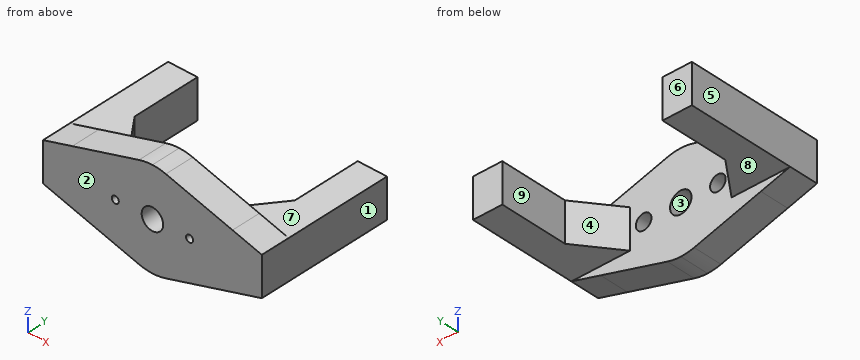
```python
from build123d import *

# Parameters (mm, degrees)
SKETCH1_R               = 25
SKETCH1_R_2             = 1.8
SKETCH1_R_3             = 5.5
BOSS_EXTRUDE1_DEPTH     = 15
SKETCH2_R               = 4
CUT_EXTRUDE1_DEPTH      = 8
SKETCH3_W               = 82
SKETCH3_H               = 50
SKETCH3_R               = 24.5
BOSS_EXTRUDE2_DEPTH     = 15
SKETCH4_W               = 15
SKETCH4_H               = 20
BOSS_EXTRUDE3_DEPTH     = 70
CUT_EXTRUDE2_DEPTH      = 94.064493766
CUT_EXTRUDE2_DEPTH_BACK = 94.064493766
BOSS_EXTRUDE4_DEPTH     = 15
CHAMFER1_SIZE           = 15
CHAMFER1_SIZE2          = 19.905672324


with BuildPart() as part:
    # Sketch1 → Boss-Extrude1 (new body)
    with BuildSketch(Plane(origin=(0, 0, 0), x_dir=(1, 0, 0), z_dir=(0, 1, 0))):
        with Locations(Location((0, 0, 0), (0, 0, 270))):
            Circle(SKETCH1_R)
        with Locations(Location((-19, 0, 0), (0, 0, 270))):
            Circle(SKETCH1_R_2, mode=Mode.SUBTRACT)
        with Locations(Location((19, 0, 0), (0, 0, 90))):
            Circle(SKETCH1_R_2, mode=Mode.SUBTRACT)
        with Locations(Location((0, 0, 0), (0, 0, 270))):
            Circle(SKETCH1_R_3, mode=Mode.SUBTRACT)
    extrude(amount=BOSS_EXTRUDE1_DEPTH)

    # Sketch2 → Cut-Extrude1 (cut)
    with BuildSketch(Plane(origin=(0, 15, 0), x_dir=(1, 0, 0), z_dir=(0, 1, 0))):
        with Locations(Location((-19, 0, 0), (0, 0, 270))):
            Circle(SKETCH2_R)
        with Locations(Location((19, 0, 0), (0, 0, 270))):
            Circle(SKETCH2_R)
    extrude(amount=-CUT_EXTRUDE1_DEPTH, mode=Mode.SUBTRACT)

    # Sketch3 → Boss-Extrude2 (add)
    with BuildSketch(Plane.XZ):
        Rectangle(SKETCH3_W, SKETCH3_H)
        Circle(SKETCH3_R, mode=Mode.SUBTRACT)
    extrude(amount=-BOSS_EXTRUDE2_DEPTH)

    # Sketch4 → Boss-Extrude3 (add)
    with BuildSketch(Plane.XZ):
        with Locations((-48.5, 0)):
            Rectangle(SKETCH4_W, SKETCH4_H)
        with Locations((48.5, 0)):
            Rectangle(SKETCH4_W, SKETCH4_H)
    extrude(amount=-BOSS_EXTRUDE3_DEPTH)

    # Sketch5 → Cut-Extrude2 (cut, two sides: drawn at the far end of the back side and taken through both)
    with BuildSketch(Plane.XZ.offset(-CUT_EXTRUDE2_DEPTH_BACK)):
        Polygon((-41, -25), (-41, -14.285834105), (-56, -10), (-56, -25), align=None)
        with BuildLine():
            ThreePointArc((-2.6e-08, -25), (-3.467621731, -24.758344039), (-6.86820572, -24.03804797))
            Line((-6.86820572, -24.03804797), (-41, -14.285834105))
            Line((-41, -14.285834105), (-41, -25))
            Line((-41, -25), (-2.6e-08, -25))
        make_face()
        Polygon((-56, 25), (-56, 10), (-41, 14.285834105), (-41, 25), align=None)
        with BuildLine():
            Line((-41, 25), (-41, 14.285834105))
            Line((-41, 14.285834105), (-6.86820572, 24.03804797))
            ThreePointArc((-6.86820572, 24.03804797), (-3.467621732, 24.758344038), (-2.8e-08, 25))
            Line((-2.8e-08, 25), (-41, 25))
        make_face()
        with BuildLine():
            Line((41, 25), (-2.8e-08, 25))
            ThreePointArc((-2.8e-08, 25), (3.467621704, 24.758344042), (6.86820572, 24.03804797))
            Line((6.86820572, 24.03804797), (41, 14.285834105))
            Line((41, 14.285834105), (41, 25))
        make_face()
        with BuildLine():
            ThreePointArc((6.86820572, -24.03804797), (3.467621705, -24.758344042), (-2.6e-08, -25))
            Line((-2.6e-08, -25), (41, -25))
            Line((41, -25), (41, -14.285834105))
            Line((41, -14.285834105), (6.86820572, -24.03804797))
        make_face()
        Polygon((41, -14.285834105), (41, -25), (56, -25), (56, -10), align=None)
        Polygon((56, 25), (41, 25), (41, 14.285834105), (56, 10), align=None)
    extrude(amount=CUT_EXTRUDE2_DEPTH + CUT_EXTRUDE2_DEPTH_BACK, mode=Mode.SUBTRACT)

    # Sketch6 → Boss-Extrude4 (add)
    with BuildSketch(Plane.XZ):
        Polygon((-56, 10), (-41, 14.285834105), (-41, -14.285834105), (-56, -10), align=None)
        Polygon((41, 14.285834105), (56, 10), (56, -10), (41, -14.285834105), align=None)
    extrude(amount=-BOSS_EXTRUDE4_DEPTH)

    # Chamfer1
    chamfer1_edges = [part.edges().sort_by_distance(p)[0] for p in [
        (-41, 15, 0),
        (41, 15, 0),
    ]]
    chamfer1_side = [part.faces().sort_by_distance(p)[0] for p in [
        (0, 15, 23.773460151),
    ]]
    chamfer(chamfer1_edges, length=CHAMFER1_SIZE, length2=CHAMFER1_SIZE2, reference=chamfer1_side[0])


solid = part.part
```
Could you check a few things on this model? Use its own coordinates, in mm. Face numbers are marked on the shaded views. A direction names the side the tool comes from. Coordinates: 2 decimals unless noted, no trailing zeros. Loops run counter-clockwise (first coordinate to the right, second up) from the corner with the lowest first, then second, coordinate; pieces in that order, holes last. Notation, with made-up numbers: M 72.5,-25 L 98.5,-25 A10 ccw 98.5,-16 Z; hole C 56.5,55 d6. An arc over 180 degrees is marked long. Put each result on its own line as item: value. Start each with the question number.
(1) I need wall thicknesses on line 1 (X direction, y = 12, z = 0); line 2 (Y direction, x = -17, z = -3.5); line 3 (X direction, y = 58, z = -6). Which ranges of each line are inside material? Lowest first, please. Write a range as from..to.
(2) Suppose I cut it at D-D on x = 19. Please give me the cut outline in (y, z).
(3) Will these pins go through, and if not, where does the flat tip stop? P1, Ø9, axis at x = -46.5, y = 51, coming from the -Z side; P2, Ø17.5, axis at x = 0, z = 0, coming from the +Y side; P3, Ø5, axis at x = 19, z = 0, coming from the +Y side; P4, Ø4, axis at x = -0.5, y = 18, coming from the -Z side.
(4) Suppose I cut it at B-B on y = 9. Please give me the cut outline in (x, z).
(5) Suppose I cut it at A-A on z = 0. Count the separate pieces of the cut face and the enclosed holes in it, then the cut area to 3 significant figures.
(6) Thinking about a two-plate mould opening in X: for the marked faces 1, 2, 3 and 4, which applies, pulls with the +X half, pulls with the -X half, needs draft (parallel to the pull), parting line crosses it, or undercut?
(7) Suppose I cut it at C-C on y = 60.5. Please give me the cut outline in (x, z).
(8) For the marked faces 5, 6, 7, 8 and 9, which set-ups out of +Z, -Z, +X, -X, +Y, -Y let a thin tool reach every point of the face, with its end or its side?
Solutions:
1. line 1: x = -56..-23, -15..-5.5, 5.5..15, 23..56
1. line 2: y = 0..15
1. line 3: x = -56..-41, 41..56
2. outline: M 0,-20.57 L 15,-20.57 L 15,-4 L 7,-4 L 7,-1.8 L 0,-1.8 Z; M 0,1.8 L 7,1.8 L 7,4 L 15,4 L 15,20.57 L 0,20.57 Z
3. P1: stops at z = -10
3. P2: stops at y = 15
3. P3: stops at y = 7
3. P4: passes through
4. outline: M -56,-10 L -6.87,-24.04 A25 ccw 6.87,-24.04 L 56,-10 L 56,10 L 6.87,24.04 A25 ccw -6.87,24.04 L -56,10 Z; hole C -19,0 d8; hole C 0,0 d11; hole C 19,0 d8
5. separate pieces: 4
5. enclosed holes: 0
5. area: 3,290 mm2
6. face 1: pulls with the +X half
6. face 2: needs draft
6. face 3: undercut
6. face 4: undercut
7. outline: M -56,-10 L -41,-10 L -41,10 L -56,10 Z; M 41,-10 L 56,-10 L 56,10 L 41,10 Z
8. face 5: +Z, -Z, -X, +Y, -Y
8. face 6: +Z, -Z, +X, -X, +Y
8. face 7: +Z, +X, -X, +Y
8. face 8: -Z, +X, -X, +Y
8. face 9: +Z, -Z, +Y
